Geometry: final body of the model. Coordinates: model frame, mm. A direction names the side the tool comes from. Coordinates: 2 decimals unless noted, no trailing zeros. Loops run counter-clockwise (first coordinate to the right, second up) from the corner with the lowest first, then second, coordinate; pieces in that order, holes last. Notation, with made-up numbers: (-16, 4) - (26, 4) arc R7 cw to (26, 13) - close; hole circle Ø2 at (65.5, 51). An arc over 180 degrees is marked (long way). Put each result on its own line as item: value. Start each with the question number.
1) Section C-C on z = 35. Output: boundary loops of the cut face in (x, y), and give its area (3 significant figures).
2) Section D-D on x = 57. Output: boundary loops of the cut face in (y, z).
3) Contact query for flat-ended pins moving along their axis: pin 1 Ø1.5 at (x, y) = (14.71, -12.7) entering from +Z; pin 2 Ø10 at (y, z) = (-20.5, 42.5) entering from +X; pin 3 Ø3.5 at (x, y) = (84.35, -50.8) entering from +Z. Output: stop coordinate, or through.
4) Material intervals for line 1 along X through (y, z) = (-50.8, 7); line 2 along X through (y, z) = (-34.5, 4); line 3 along X through (y, z) = (-16, 18.5), sorted ascending. Write a range as from..to.
5) Section B-B on y = -27.5. Output: boundary loops of the cut face in (x, z).
6) Reachability of faces 1 (the flat face through (15, -34, 25.4)), 2 (the flat face through (30.036, -31, 19)), 3 (the flat face through (99.06, -31, 13)) from +Z, -Z, +X, -X, +Y, -Y: full face, straight path, thin tool, end or side. Return the list, or none.
7) Draft query along X for faces 4 (the cylindrical face through (91.82, -32.19, 43.16)), 5 (the flat face through (49, -63.5, 43)), 6 (the flat face through (84, -51, 25.4)). Return one class per face: +X half, -X half, draft (parallel to the pull), parting line (faces both ways), or undercut.
8) Section A-A on z = 13. Output: boundary loops of the cut face in (x, y), and give its area (3 significant figures).
```python
from build123d import *

# Parameters (mm, degrees)
F1_DEPTH = 63.5
F2_R     = 25.4
F3_R     = 1.3335
F3_R_2   = 1.27
F4_DEPTH = 25.4


with BuildPart() as f1:
    # F0 (on Front) → F1 (new body)
    with BuildSketch(Plane.XZ):
        Polygon((0, 50.8), (0, 0), (30.0355, 0), (30.0355, 38.1762), (69.0245, 38.1762), (69.0245, 0), (99.06, 0), (99.06, 50.8), align=None)
    extrude(amount=F1_DEPTH)

    # F2
    f2_edges = [f1.edges().sort_by_distance(p)[0] for p in [
        (99.06, -31.75, 50.8),
        (0, -31.75, 50.8),
    ]]
    fillet(f2_edges, radius=F2_R)

    # F3 (on face) → F4 (cut)
    with BuildSketch(Plane(origin=(0, 0, 0), x_dir=(1, 0, 0), z_dir=(0, 0, -1))):
        with Locations((14.7066, 34.29)):
            Circle(F3_R)
        with Locations((84.3534, 34.29)):
            Circle(F3_R)
        with Locations((14.7066, 12.7)):
            Circle(F3_R_2)
        with Locations((84.3534, 12.7)):
            Circle(F3_R_2)
        with Locations((84.3534, 50.8)):
            Circle(F3_R_2)
        with Locations((14.7066, 50.8)):
            Circle(F3_R_2)
    extrude(amount=-F4_DEPTH, mode=Mode.SUBTRACT)


solid = f1.part
```
Answer block:
1. outline: (1.88, -63.5) - (30.04, -63.5) - (30.04, 0) - (1.88, 0) - close; (69.02, -63.5) - (97.18, -63.5) - (97.18, 0) - (69.02, 0) - close
1. area: 3,580 mm²
2. outline: (-63.5, 38.18) - (0, 38.18) - (0, 50.8) - (-63.5, 50.8) - close
3. pin 1: stops at z = 48.77
3. pin 2: stops at x = 95.99
3. pin 3: stops at z = 49.17
4. line 1: x = 0..13.44, 15.98..30.04, 69.02..83.08, 85.62..99.06
4. line 2: x = 0..13.39, 16.02..30.04, 69.02..83.04, 85.67..99.06
4. line 3: x = 0..30.04, 69.02..99.06
5. outline: (0, 0) - (30.04, 0) - (30.04, 38.18) - (69.02, 38.18) - (69.02, 0) - (99.06, 0) - (99.06, 25.4) arc R25.4 ccw to (73.66, 50.8) - (25.4, 50.8) arc R25.4 ccw to (0, 25.4) - close
6. face 1: -Z
6. face 2: -Z, +Y, -Y
6. face 3: +Z, -Z, +X, +Y, -Y
7. face 4: +X half
7. face 5: draft
7. face 6: undercut
8. outline: (0, -63.5) - (30.04, -63.5) - (30.04, 0) - (0, 0) - close; (69.02, -63.5) - (99.06, -63.5) - (99.06, 0) - (69.02, 0) - close; hole circle Ø2.67 at (14.71, -34.29); hole circle Ø2.54 at (14.71, -50.8); hole circle Ø2.54 at (14.71, -12.7); hole circle Ø2.67 at (84.35, -34.29); hole circle Ø2.54 at (84.35, -50.8); hole circle Ø2.54 at (84.35, -12.7)
8. area: 3,780 mm²
